from build123d import *

# Parameters (mm, degrees)
SKETCH_1_R          = 0.9
EXTRUDE_1_DEPTH     = 1.5
FILLET_1_R          = 3
SKETCH_2_R          = 0.9
CUT_EXTRUDE_1_DEPTH = 10


with BuildPart() as part:
    # 草图1 → 凸台-拉伸1 (new body)
    with BuildSketch(Plane(origin=(0, 0, 0), x_dir=(0, 0, -1), z_dir=(1, 0, 0))):
        with BuildLine():
            Line((-14.5, 0), (-14.5, 16))
            Line((-14.5, 16), (0, 24.133548193))
            Line((0, 24.133548193), (14.5, 16))
            Line((14.5, 16), (14.5, 0))
            ThreePointArc((14.5, 0), (17, -2.5), (19.5, 0))
            Line((19.5, 0), (19.5, 18.928231824))
            Line((19.5, 18.928231824), (1.22305902, 29.180395981))
            ThreePointArc((1.22305902, 29.180395981), (0, 29.5), (-1.22305902, 29.180395981))
            Line((-1.22305902, 29.180395981), (-19.5, 18.928231824))
            Line((-19.5, 18.928231824), (-19.5, 0))
            ThreePointArc((-19.5, 0), (-17, -2.5), (-14.5, 0))
        make_face()
        with Locations((-17, 0)):
            Circle(SKETCH_1_R, mode=Mode.SUBTRACT)
        with Locations(Location((17, 0, 0), (0, 0, 180))):  # turned: the seam where the file's is
            Circle(SKETCH_1_R, mode=Mode.SUBTRACT)
        with Locations((0, 27)):
            Circle(SKETCH_1_R, mode=Mode.SUBTRACT)
    extrude(amount=EXTRUDE_1_DEPTH)

    # 圆角1
    fillet_1_edges = [part.edges().sort_by_distance(p)[0] for p in [
        (0.75, 18.928231824, 19.5),
        (0.75, 18.928231824, -19.5),
        (0.75, 16, -14.5),
        (0.75, 24.133548193, 0),
        (0.75, 16, 14.5),
    ]]
    fillet(fillet_1_edges, radius=FILLET_1_R)

    # 草图2 → 切除-拉伸1 (cut)
    with BuildSketch(Plane(origin=(1.5, 0, 0), x_dir=(0, 0, -1), z_dir=(1, 0, 0))):
        with Locations((-17, 16.5)):
            Circle(SKETCH_2_R)
        with Locations((-17, 8.25)):
            Circle(SKETCH_2_R)
        with Locations((17, 8.25)):
            Circle(SKETCH_2_R)
        with Locations((17, 16.5)):
            Circle(SKETCH_2_R)
    extrude(amount=-CUT_EXTRUDE_1_DEPTH, mode=Mode.SUBTRACT)

    # 草图3 → M2 平头机械螺钉的锥形沉头孔1 (revolve, cut)
    with BuildSketch(Plane(origin=(1.5, 27, 0), x_dir=(0, 0, -1), z_dir=(0, 1, 0))):
        Polygon((0, 0), (0, 1.5), (0.85, 1.5), (0.85, 1.2), (2.05, 0), align=None)
    revolve(axis=Axis((7.85, 27, 0), (-1, 0, 0)), mode=Mode.SUBTRACT)


solid = part.part
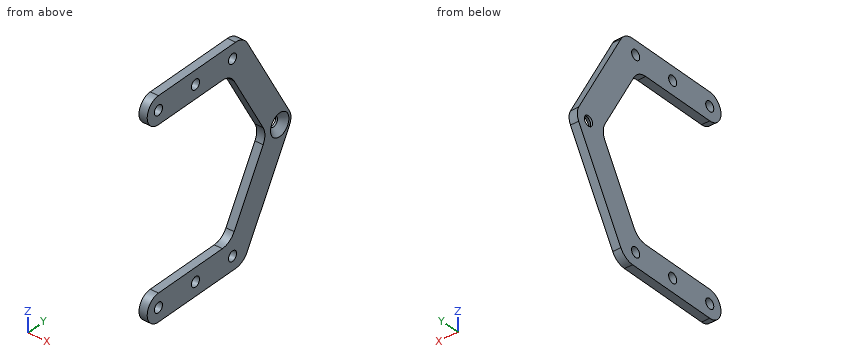
Design review of the part built by this model. Coordinates are the model's own, in mm. Round coordinates to 2 decimals unless told otherwise and drop trailing zeros. Loops run counter-clockwise (first coordinate to the right, second up) from the corner with the lowest first, then second, coordinate; pieces in that order, holes last. Notation, with made-up numbers: (9.25, -37) - (54.25, -37) arc R28 cw to (54.25, -8) - close; hole circle Ø3 at (16, 9). An arc over 180 degrees is marked (long way). One line per question, with ' | ' between items.
1. We need section D-D, the plane z = -17. State the section outline as (x, y) points.
Results are:
outline: (0, -2.5) - (1.5, -2.5) - (1.5, -0.9) - (0, -0.9) - close; (0, 0.9) - (1.5, 0.9) - (1.5, 7.35) - (0, 7.35) - close; (0, 9.15) - (1.5, 9.15) - (1.5, 15.6) - (0, 15.6) - close; (0, 17.4) - (1.5, 17.4) - (1.5, 20.33) - (0, 20.33) - close
2. We need section A-A, the plane z = 0. State the section outline as (x, y) points.
Results are:
outline: (0, 23.69) - (1.5, 23.69) - (1.5, 24.95) - (0.35, 26.1) - (0, 26.1) - close; (0, 27.9) - (0.35, 27.9) - (1.5, 29.05) - (1.5, 29.5) - (0, 29.5) - close
3. For L1, parallel to Z at x = 1.2, y = 7; L2, parallel to Y at x = 0.1, z = 0; L3, parallel to Y at x = 0.9, z = -17, list the stretches that pass through material, from the lowest coordinate up. Write a range as [from, to].
Results are:
L1: z = [-19.5, -14.5], [14.5, 19.5] | L2: y = [23.69, 26.1], [27.9, 29.5] | L3: y = [-2.5, -0.9], [0.9, 7.35], [9.15, 15.6], [17.4, 20.33]
4. We need section B-B, the plane y = 8.25. State the section outline as (x, z) points.
Results are:
outline: (0, -19.5) - (1.5, -19.5) - (1.5, -17.9) - (0, -17.9) - close; (0, -16.1) - (1.5, -16.1) - (1.5, -14.5) - (0, -14.5) - close; (0, 14.5) - (1.5, 14.5) - (1.5, 16.1) - (0, 16.1) - close; (0, 17.9) - (1.5, 17.9) - (1.5, 19.5) - (0, 19.5) - close
5. We need section C-C, the plane y = 27. State the section outline as (x, z) points.
Results are:
outline: (0, -5.11) - (1.5, -5.11) - (1.5, -2.05) - (0.35, -0.9) - (0, -0.9) - close; (0, 0.9) - (0.35, 0.9) - (1.5, 2.05) - (1.5, 5.11) - (0, 5.11) - close
